Here's how the part is built. I have some questions about the finished solid (model axes, mm). A direction names the side the tool comes from. Give positions to 0.01 mm unless a question says otherwise; leave off trailing zeros. Loops run counter-clockwise (first coordinate to the right, second up) from the corner with the lowest first, then second, coordinate; pieces in that order, holes last. Notation, with made-up numbers: (41, 23.5) - (92, 23.5) arc R16 ccw to (92, 44.5) - close; hole circle Ø2 at (82, 48.25). An arc over 180 degrees is marked (long way). Use a Markdown table: item, result.
from build123d import *

# Parameters (mm, degrees)
F0_W      = 203.2
F0_H      = 127
F1_DEPTH  = 127
F3_DEPTH  = 101.6
F4_DEPTH  = 50.8
F5_SIZE2  = 101.6
F5_SIZE   = 76.2
F6_R      = 5.08
F8_DEPTH  = 76.2
F9_R      = 19.05
F10_DEPTH = 127
F12_D     = 6.35


with BuildPart() as f1:
    # F0 (on Front) → F1 (new body)
    with BuildSketch(Plane.XZ):
        with Locations((2.3381854308, 0)):
            Rectangle(F0_W, F0_H)
    extrude(amount=F1_DEPTH)

    # F2 (on face) → F3 (cut)
    with BuildSketch(Plane.XZ.offset(127)):
        Polygon((-35.7618145692, 0), (-35.7618145692, -63.5), (103.9381854308, -63.5), (103.9381854308, 63.5), (2.3381854308, 63.5), (2.3381854308, 0), align=None)
    extrude(amount=-F3_DEPTH, mode=Mode.SUBTRACT)

    # F4 (add): a face of the model
    f4_faces = [f1.faces().sort_by_distance(p)[0] for p in [
        (42.1092380623, -25.4, -5.0131578947),
    ]]
    extrude(f4_faces, amount=F4_DEPTH)

    # F5
    f5_edges = [f1.edges().sort_by_distance(p)[0] for p in [
        (103.938185, -38.1, 63.5),
    ]]
    f5_side = f1.faces().sort_by_distance((-10.361815, -53.975, 63.5))[0]
    chamfer(f5_edges, length=F5_SIZE, length2=F5_SIZE2, reference=f5_side)

    # F6
    f6_edges = [f1.edges().sort_by_distance(p)[0] for p in [
        (-67.511815, -127, -63.5),
        (2.338185, -101.6, 0),
        (-35.761815, -101.6, -63.5),
        (-99.261815, -63.5, 63.5),
        (2.338185, -101.6, 63.5),
        (15.038185, -76.2, 63.5),
        (65.838185, -76.2, 12.7),
        (-16.711815, -127, 0),
        (103.938185, -38.1, -63.5),
        (-35.761815, 0, 63.5),
        (65.838185, 0, 12.7),
        (34.088185, -76.2, -63.5),
        (-48.461815, -127, 63.5),
        (27.738185, -38.1, 63.5),
        (103.938185, -38.1, -38.1),
        (-35.761815, -76.2, -31.75),
        (-99.261815, 0, 0),
        (-16.711815, -76.2, 0),
        (2.338185, 0, -63.5),
        (-99.261815, -127, 0),
        (-99.261815, -63.5, -63.5),
        (-35.761815, -101.6, 0),
        (2.338185, -76.2, 31.75),
        (2.338185, -127, 31.75),
        (-35.761815, -127, -31.75),
        (103.938185, 0, -50.8),
        (103.938185, -76.2, -50.8),
    ]]
    fillet(f6_edges, radius=F6_R)

    # F7 (on face) → F8 (cut, through all)
    with BuildSketch(Plane.XZ.offset(76.2)):
        with BuildLine():
            Line((19.7116794232, -18.8833934691), (34.9488621098, -18.5903682534))
            ThreePointArc((34.9488621098, -18.5903682534), (8.7301641023, -8.3162783823), (20.0047046389, -34.1205761556))
            Line((20.0047046389, -34.1205761556), (19.7116794232, -18.8833934691))
        make_face()
        with BuildLine():
            ThreePointArc((20.0047046389, -34.1205761556), (30.5910935684, -29.5555979207), (34.9516794232, -18.8833934691))
            ThreePointArc((34.9516794232, -18.8833934691), (34.9509750786, -18.7368740896), (34.9488621098, -18.5903682534))
            Line((34.9488621098, -18.5903682534), (19.7116794232, -18.8833934691))
            Line((19.7116794232, -18.8833934691), (20.0047046389, -34.1205761556))
        make_face()
    extrude(amount=-F8_DEPTH, mode=Mode.SUBTRACT)

    # F9 (on face) → F10 (cut, through all)
    with BuildSketch(Plane.XY.offset(63.5)):
        with Locations((-61.6576299071, -73.365047574)):
            Circle(F9_R)
    extrude(amount=-F10_DEPTH, mode=Mode.SUBTRACT)

    # F12 (through all)
    with Locations(Plane.XY.offset(63.5)):
        with Locations((-44.0687574446, -20.4515326768), (-44.0687574446, -36.8853211403), (-20.3539002687, -20.4515326768), (-20.3539002687, -36.8853211403)):
            Hole(F12_D / 2)


solid = f1.part
(1) Suppose I cut it at B-B on x = -58.5. Write out the boundary of the cut face in (y, z), plus the area to 3 significant figures.
A:
| item | result |
|---|---|
| outline | (-127, -58.42) arc R5.08 ccw to (-121.92, -63.5) - (-92.15, -63.5) - (-92.15, 63.5) - (-121.92, 63.5) arc R5.08 ccw to (-127, 58.42) - close; (-54.58, -63.5) - (-5.08, -63.5) arc R5.08 ccw to (0, -58.42) - (0, 58.42) arc R5.08 ccw to (-5.08, 63.5) - (-54.58, 63.5) - close |
| area | 11,300 mm2 |
(2) Suppose I cut it at D-D on y = -114. Write out the boundary of the cut face in (x, z).
A:
| item | result |
|---|---|
| outline | (-99.26, -58.42) arc R5.08 ccw to (-94.18, -63.5) - (-40.84, -63.5) arc R5.08 ccw to (-35.76, -58.42) - (-35.76, -5.08) arc R5.08 cw to (-30.68, 0) - (-2.74, 0) arc R5.08 ccw to (2.34, 5.08) - (2.34, 58.42) arc R5.08 ccw to (-2.74, 63.5) - (-94.18, 63.5) arc R5.08 ccw to (-99.26, 58.42) - close |
(3) We'd pull the mould along X, two halves only. Please class faces 1 (the face through (102.49, -1.53, -48.98)), 2 (the face through (-20, 0, 1)), 3 (the face through (-19.67, -23.55, -0.89)): pulls with the +X half, pulls with the -X half, needs draft (parallel to the pull), parting line crosses it, or undercut.
A:
| item | result |
|---|---|
| face 1 | pulls with the +X half |
| face 2 | needs draft |
| face 3 | undercut |
(4) If I drill on line 1 (Y direction, x = 51, z = -43); line 2 (X direction, y = -34, z = -37.5); line 3 (X direction, y = -120.5, z = -27.5), over which ranges is the centre line in solid material (lowest first)?
A:
| item | result |
|---|---|
| line 1 | -76.2 to 0 |
| line 2 | -99.26 to -45.39, -42.74 to -21.68, -19.03 to 103.39 |
| line 3 | -99.26 to -35.76 |
(5) Will these pins go through, and if not, where does the flat tip stop? pin 1 (5 mm diameter, centred on x = -44.07, y = -20.45, fed in from -Z); pin 2 (1 mm diameter, centred on y = -27.5, z = 21, fed in from +X); pin 3 (3 mm diameter, centred on x = 36.5, z = 49.5, fed in from -Y); pin 4 (12 mm diameter, centred on y = -106, z = 44.5, fed in from +X).
A:
| item | result |
|---|---|
| pin 1 | through |
| pin 2 | x = 59.99 |
| pin 3 | y = -75.7 |
| pin 4 | x = 2.34 |
(6) Suppose I cut it at A-A on y = -45. Write out the boundary of the cut face in (x, z), plus the area to 3 significant figures.
A:
| item | result |
|---|---|
| outline | (-99.26, -58.42) arc R5.08 ccw to (-94.18, -63.5) - (98.86, -63.5) arc R5.08 ccw to (103.94, -58.42) - (103.94, -39.79) arc R5.08 ccw to (102.92, -36.75) - (29.26, 61.47) arc R5.08 ccw to (25.2, 63.5) - (-94.18, 63.5) arc R5.08 ccw to (-99.26, 58.42) - close; hole circle Ø30.48 at (19.71, -18.88) |
| area | 21,200 mm2 |
(7) On a 3-axis mill with a long thin cutter (end or side, diameter ignored), from which of +Z, -Z, +X, -X, +Y, -Y can I reach the whole of each face in a straight line? I mean faces 4 (the face through (0.81, -101.32, 62.05)), 5 (the face through (-43.38, -23.55, -0.89)), 6 (the face through (48, -76.2, -12)). Say none if no direction works.
A:
| item | result |
|---|---|
| face 4 | +Z, +X, -Y |
| face 5 | +Z, -Z |
| face 6 | -Z, +X, -Y |
(8) Suppose I cut it at C-C on y = -67. Write out the boundary of the cut face in (x, z).
A:
| item | result |
|---|---|
| outline | (-99.26, -58.42) arc R5.08 ccw to (-94.18, -63.5) - (-79.61, -63.5) - (-79.61, 63.5) - (-94.18, 63.5) arc R5.08 ccw to (-99.26, 58.42) - close; (-43.7, -63.5) - (98.86, -63.5) arc R5.08 ccw to (103.94, -58.42) - (103.94, -39.79) arc R5.08 ccw to (102.92, -36.75) - (29.26, 61.47) arc R5.08 ccw to (25.2, 63.5) - (-43.7, 63.5) - close; hole circle Ø30.48 at (19.71, -18.88) |
